Drawing for the job (mm, zero at the part's lowest x, y, z). A direction names the side the tool comes from. Give positions to 0.01 mm unless a question says otherwise; leave off trailing zeros. Loops run counter-clockwise (first coordinate to the right, second up) from the corner with the lowest first, then second, coordinate; pieces in that order, holes last. Notation, with made-up numbers: (6, -37.75) -> (45, -37.75) arc R8 cw to (45, -29.75) -> close; hole circle Ø3 at (53, -29). An arc over 180 degrees is marked (long way). Use CSV: the item, a comma, the result in double quotes. Start each with the question number.
(1) Cut at C-C on y = 14.5. Write the cut outline in (x, z).
(2) Flat gauge pins, fed straight in: pin 1 (3 mm diameter, centred on x = 28, z = 4.5, fed in from -Y); pin 2 (6 mm diameter, centred on x = 28.5, y = 17, fed in from -Z); pin 3 (3 mm diameter, centred on x = 30, z = 10, fed in from +Y). Where does each tip first touch, or does it go through?
(3) 3-axis set-ups, long thin cutter, end or side, ignore diameter. For the marked faces 4 and 5: which of +Z, -Z, +X, -X, +Y, -Y reach the whole face in a straight line?
(4) Cut at D-D on z = 23.5. Write the cut outline in (x, y).
(5) Pull direction X, two halves, no side cores. Call the marked faces 1, 2 and 3: pulls with the +X half, pulls with the -X half, needs draft (parallel to the pull), parting line crosses it, or undercut.
(6) Cut at A-A on x = 10. Write the cut outline in (y, z), then the cut area to 3 significant figures.
(7) Cut at B-B on z = 10. Write the cut outline in (x, y), then the cut area to 3 significant figures.
(8) Drill centre lines: probe 1 along Z at (x, y) = (10, 2); probe 2 along X at (y, z) = (2, 10.25); probe 3 along Z at (x, y) = (12, 13.75). Where is each one in solid material? Low to high.
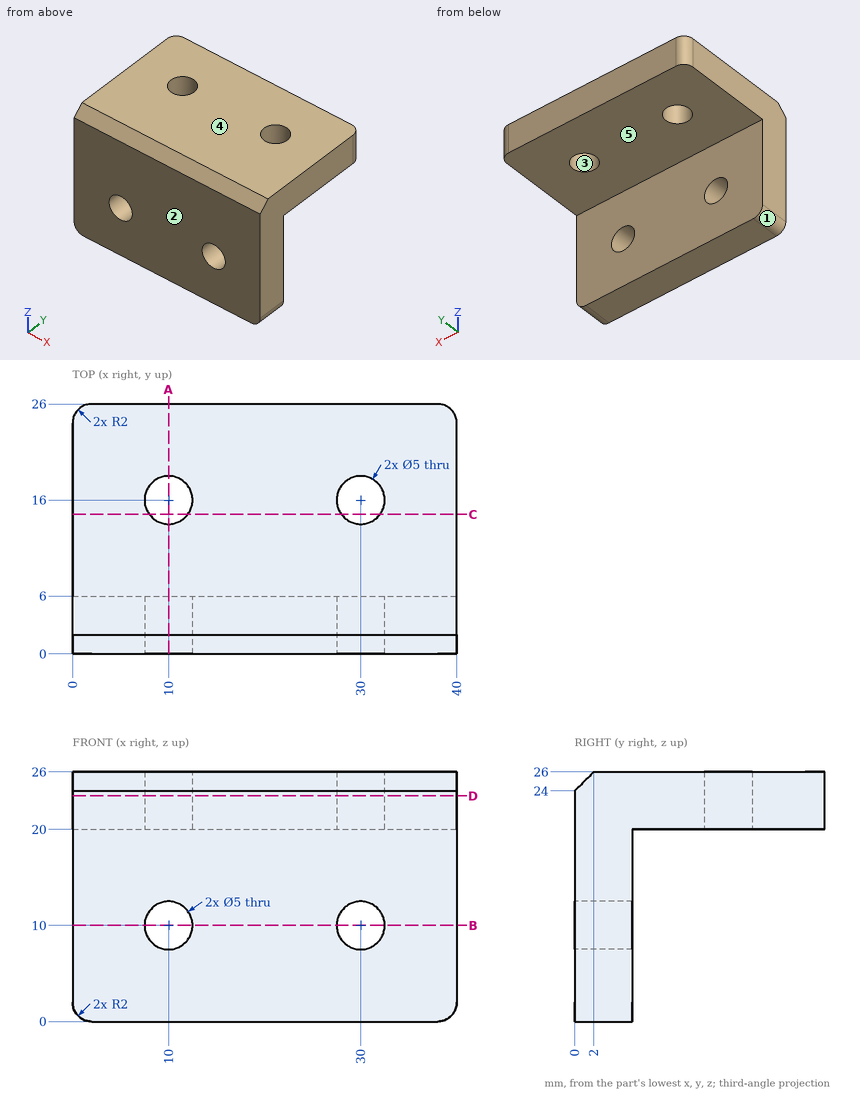
Check result:
1,outline,"(0, 20) -> (8, 20) -> (8, 26) -> (0, 26) -> close; (12, 20) -> (28, 20) -> (28, 26) -> (12, 26) -> close; (32, 20) -> (40, 20) -> (40, 26) -> (32, 26) -> close"
2,pin 1,"y = 0"
2,pin 2,"z = 20"
2,pin 3,"through"
3,face 4,"+Z, +X, -X, +Y, -Y"
3,face 5,"-Z, +X, -X, +Y"
4,outline,"(0, 0) -> (40, 0) -> (40, 24) arc R2 ccw to (38, 26) -> (2, 26) arc R2 ccw to (0, 24) -> close; hole circle Ø5 at (10, 16); hole circle Ø5 at (30, 16)"
5,face 1,"pulls with the -X half"
5,face 2,"needs draft"
5,face 3,"undercut"
6,outline,"(0, 0) -> (6, 0) -> (6, 7.5) -> (0, 7.5) -> close; (0, 12.5) -> (6, 12.5) -> (6, 20) -> (13.5, 20) -> (13.5, 26) -> (2, 26) -> (0, 24) -> close; (18.5, 20) -> (26, 20) -> (26, 26) -> (18.5, 26) -> close"
6,area,"214 mm²"
7,outline,"(0, 0) -> (7.5, 0) -> (7.5, 6) -> (0, 6) -> close; (12.5, 0) -> (27.5, 0) -> (27.5, 6) -> (12.5, 6) -> close; (32.5, 0) -> (40, 0) -> (40, 6) -> (32.5, 6) -> close"
7,area,"180 mm²"
8,probe 1,"0 to 7.5, 12.5 to 26"
8,probe 2,"0 to 7.51, 12.49 to 27.51, 32.49 to 40"
8,probe 3,"20 to 26"
